CAD build for the part. Positions are in the model's coordinates, mm. Face numbers are marked on the shaded views. A direction names the side the tool comes from. Round coordinates to 2 decimals unless told otherwise and drop trailing zeros. Loops run counter-clockwise (first coordinate to the right, second up) from the corner with the lowest first, then second, coordinate; pieces in that order, holes last.
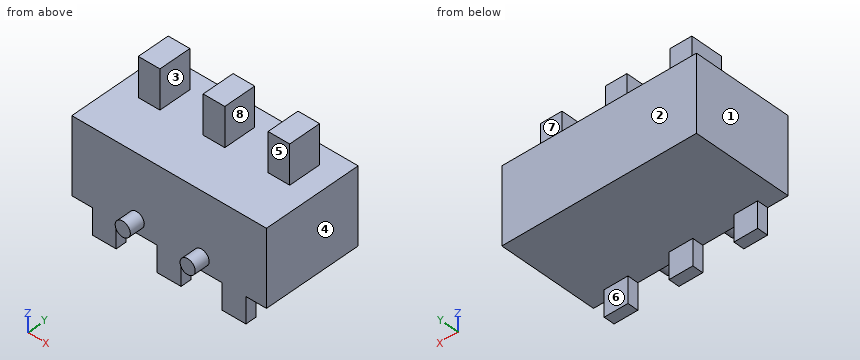
from build123d import *

# Parameters (mm, degrees)
SKETCH1_W           = 9
SKETCH1_H           = 3.5
BOSS_EXTRUDE1_DEPTH = 4.6
SKETCH2_W           = 1
SKETCH2_H           = 1.5
BOSS_EXTRUDE2_DEPTH = 1.8
LPATTERN1_COUNT     = 2
LPATTERN1_PITCH     = 3
LPATTERN1_COL_COUNT = 2
LPATTERN1_COL_PITCH = 3
SKETCH5_R           = 0.35
BOSS_EXTRUDE4_DEPTH = 0.7
SKETCH3_W           = 1.1
SKETCH3_H           = 0.5
BOSS_EXTRUDE3_DEPTH = 1.2
LPATTERN2_COUNT     = 2
LPATTERN2_PITCH     = 3
LPATTERN2_COL_COUNT = 2
LPATTERN2_COL_PITCH = 3


with BuildPart() as part:
    # Sketch1 → Boss-Extrude1 (new body)
    with BuildSketch(Plane(origin=(0, 0, 0), x_dir=(1, 0, 0), z_dir=(0, 1, 0))):
        Rectangle(SKETCH1_W, SKETCH1_H)
    extrude(amount=BOSS_EXTRUDE1_DEPTH)

    # Sketch2 → Boss-Extrude2 (add)
    with BuildSketch(Plane.XY.offset(1.75)):
        with Locations((0, 3)):
            Rectangle(SKETCH2_W, SKETCH2_H)
    boss_extrude2 = extrude(amount=BOSS_EXTRUDE2_DEPTH)

    # LPattern1: Boss-Extrude2 ×2
    with Locations(*[(i * LPATTERN1_PITCH, 0, 0) for i in range(1, LPATTERN1_COUNT)]):
        add(boss_extrude2)

    # LPattern1 col: Boss-Extrude2 ×2
    with Locations(*[(-i * LPATTERN1_COL_PITCH, 0, 0) for i in range(1, LPATTERN1_COL_COUNT)]):
        add(boss_extrude2)

    # Sketch5 → Boss-Extrude4 (add)
    with BuildSketch(Plane.XZ):
        with Locations((-1.5, -1.15)):
            Circle(SKETCH5_R)
        with Locations((1.5, -1.15)):
            Circle(SKETCH5_R)
    extrude(amount=BOSS_EXTRUDE4_DEPTH)

    # Sketch3 → Boss-Extrude3 (add)
    with BuildSketch(Plane(origin=(0, 0, -1.75), x_dir=(-1, 0, 0), z_dir=(0, 0, -1))):
        with Locations((0, 0.25)):
            Rectangle(SKETCH3_W, SKETCH3_H)
    boss_extrude3 = extrude(amount=BOSS_EXTRUDE3_DEPTH)

    # LPattern2: Boss-Extrude3 ×2
    with Locations(*[(i * LPATTERN2_PITCH, 0, 0) for i in range(1, LPATTERN2_COUNT)]):
        add(boss_extrude3)

    # LPattern2 col: Boss-Extrude3 ×2
    with Locations(*[(-i * LPATTERN2_COL_PITCH, 0, 0) for i in range(1, LPATTERN2_COL_COUNT)]):
        add(boss_extrude3)


solid = part.part
Item 1: Cut at A-A (z = 2.5). List the corners of the cut face in (x, y).
Verdict:
outline: (-3.5, 2.25) - (-2.5, 2.25) - (-2.5, 3.75) - (-3.5, 3.75) - close; (-0.5, 2.25) - (0.5, 2.25) - (0.5, 3.75) - (-0.5, 3.75) - close; (2.5, 2.25) - (3.5, 2.25) - (3.5, 3.75) - (2.5, 3.75) - close
Item 2: Cut at C-C (y = 0.15). List the corners of the cut face in (x, z), plus the area to 3 significant figures.
Verdict:
outline: (-4.5, -1.75) - (-3.55, -1.75) - (-3.55, -2.95) - (-2.45, -2.95) - (-2.45, -1.75) - (-0.55, -1.75) - (-0.55, -2.95) - (0.55, -2.95) - (0.55, -1.75) - (2.45, -1.75) - (2.45, -2.95) - (3.55, -2.95) - (3.55, -1.75) - (4.5, -1.75) - (4.5, 1.75) - (-4.5, 1.75) - close
area: 35.5 mm2
Item 3: 3-axis set-ups, long thin cutter, end or side, ignore diameter. For the marked faces 5, 6, 7 and 8: which of +Z, -Z, +X, -X, +Y, -Y reach the whole face in a straight line?
Verdict:
face 5: +Z, +X, -X, -Y
face 6: -Z, +X, -X, +Y
face 7: +Z, +X, -X, +Y
face 8: +Z, +Y, -Y
Item 4: Cut at B-B (x = -1.5). List the corners of the cut face in (y, z), plus the area to 3 significant figures.
Verdict:
outline: (-0.7, -1.5) - (0, -1.5) - (0, -1.75) - (4.6, -1.75) - (4.6, 1.75) - (0, 1.75) - (0, -0.8) - (-0.7, -0.8) - close
area: 16.6 mm2
Item 5: Wall check: L1, parallel to X at y = 0.3, z = -2; L2, parallel to Z at x = -3, y = 3.5; L3, parallel to Y at x = 2.5, z = 0. Give the ranges that are in metal, low to high.
Verdict:
L1: x = -3.55 to -2.45, -0.55 to 0.55, 2.45 to 3.55
L2: z = -1.75 to 3.55
L3: y = 0 to 4.6
Item 6: Mould opens along X. For the marked faces 1, 2, 3 and 4 say: released by +X, released by -X, zero draft, split by the parting line, or undercut.
Verdict:
face 1: released by -X
face 2: zero draft
face 3: undercut
face 4: released by +X
Item 7: Flat gauge pins, fed straight in: P1, Ø0.8, axis at x = 0, z = 2.5, coming from the -Y side; P2, Ø3, axis at x = -2, y = 2.5, coming from the -Z side; P3, Ø0.5, axis at x = -3, z = 2.5, coming from the +Y side. Where does each tip first touch, or does it go through?
Verdict:
P1: stops at y = 2.25
P2: stops at z = -1.75
P3: stops at y = 3.75
Item 8: Cut at D-D (z = -1.15). List the corners of the cut face in (x, y).
Verdict:
outline: (-4.5, 0) - (-1.85, 0) - (-1.85, -0.7) - (-1.15, -0.7) - (-1.15, 0) - (1.15, 0) - (1.15, -0.7) - (1.85, -0.7) - (1.85, 0) - (4.5, 0) - (4.5, 4.6) - (-4.5, 4.6) - close
